Autodesk Inventor part; units mm, degrees
ref_plane "YZ Plane" through (0, 0, 0) normal (1, 0, 0) x (0, 1, 0)
ref_plane "XZ Plane" through (0, 0, 0) normal (0, 1, 0) x (-1, 0, 0)
ref_plane "XY Plane" through (0, 0, 0) normal (0, 0, 1) x (1, 0, 0)
sketch "Эскиз1" plane through (0, 0, 0) normal (0, 0, 1) x (1, 0, 0)
  circle A0 centre (0, 0) radius 11
  circle A1 centre (0, 0) radius 7.5
  circle A2 centre (-7.5, 0) radius 1.5
  circle A3 centre (0, -7.5) radius 1.5
  circle A4 centre (7.5, 0) radius 1.5
  circle A5 centre (0, 7.5) radius 1.5
  circle A6 centre (0, 0) radius 3
  dimension "d1" = 15
  dimension "d0" = 22
  dimension "d2" = 3
  dimension "d5" = 360
  dimension "d7" = 6
extrude "Выдавливание1" add sketch "Эскиз1" along normal blind 3 contours A0 | A4 A1 A3 A2 A5
sketch "Эскиз2" plane through (0, 0, 3) normal (0, 0, 1) x (1, 0, 0)
  circle A0 centre (0, 0) radius 4.5
  circle A1 centre (0, 0) radius 11
  circle A2 centre (0, 7.5) radius 1.5
  circle A3 centre (-7.5, 0) radius 1.5
  circle A4 centre (0, -7.5) radius 1.5
  circle A5 centre (0, 0) radius 3
  circle A6 centre (7.5, 0) radius 1.5
  dimension "d10" = 9
extrude "Выдавливание2" add sketch "Эскиз2" along normal blind 9 contours A0
fillet "Сопряжение1" radius 0.5 2 edges at (-11, 0, 3) (-4.5, 0, 3)
chamfer "Фаска1" distance 0.5 angle 45 2 edges at (-4.5, 0, 12) (-3, 0, 12)
properties part number "МУФТА НА ВАЛ"
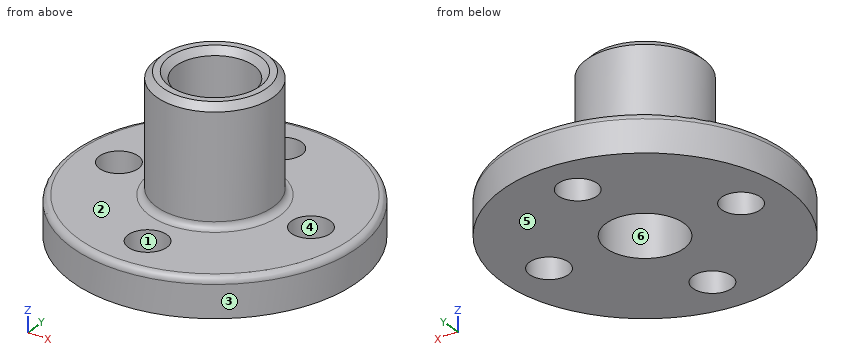
Check sheet for the modelled part. Datum: model origin and axes. Units: mm. Face numbers are marked on the shaded views. A direction names the side the tool comes from. Round coordinates to 2 decimals unless told otherwise and drop trailing zeros. Order: outer loops, then holes, each group sorted by start corner. A loop starts at its lowest first (then second) coordinate and runs counter-clockwise, first axis right, second up. Notation, with made-up numbers: (4.5, 43.25) -> (58.5, 43.25) arc R30 cw to (58.5, 69.25) -> close; hole circle Ø10 at (62.5, 43). An arc over 180 degrees is marked (long way). Use CSV: the item, a comma, the result in double quotes.
(1) Cross-section at A-A (x = 0). Record the boundary of the cut face in (y, z), and give its area (3 significant figures).
Worked out:
outline,"(-11, 0) -> (-9, 0) -> (-9, 3) -> (-10.5, 3) arc R0.5 ccw to (-11, 2.5) -> close; (-6, 0) -> (-3, 0) -> (-3, 11.5) -> (-3.5, 12) -> (-4, 12) -> (-4.5, 11.5) -> (-4.5, 3.5) arc R0.5 cw to (-5, 3) -> (-6, 3) -> close; (3, 0) -> (6, 0) -> (6, 3) -> (5, 3) arc R0.5 cw to (4.5, 3.5) -> (4.5, 11.5) -> (4, 12) -> (3.5, 12) -> (3, 11.5) -> close; (9, 0) -> (11, 0) -> (11, 2.5) arc R0.5 ccw to (10.5, 3) -> (9, 3) -> close"
area,"56.5 mm²"
(2) Draft check along Y on the marked faces 3, 4, 5 and 6. Enter one of: pulls with the +Y half, pulls with the -Y half, needs draft (parallel to the pull), parting line crosses it, or undercut.
Worked out:
face 3,"parting line crosses it"
face 4,"undercut"
face 5,"needs draft"
face 6,"undercut"
(3) Tool access check on the marked faces 1 and 2. Record the directions out of +Z, -Z, +X, -X, +Y, -Y that give a thin tool (end or side, any length) a straight path to the whole face; none if there is none.
Worked out:
face 1,"+Z, -Z"
face 2,"+Z"
(4) Material ranges on line 1 along Y through (x, z) = (0, 2.05); line 2 along Y through (x, z) = (0, 8.5); line 3 along Z through (x, y) = (-8.5, 4.75), recorded low to high. Write a range as from..to.
Worked out:
line 1,"-11..-9, -6..-3, 3..6, 9..11"
line 2,"-4.5..-3, 3..4.5"
line 3,"0..3"
(5) Depth check by flat-ended pin: pin 1 (4 mm diameter, centred on x = 0, y = 7.5, fed in from +Z); pin 2 (2 mm diameter, centred on x = 1, z = 7.5, fed in from +Y); pin 3 (2 mm diameter, centred on y = 3, z = 7.5, fed in from -X). Enter the tip coordinate at first touch or a pass-through.
Worked out:
pin 1,"z = 3"
pin 2,"y = 4.5"
pin 3,"x = -4.03"
(6) Cross-section at B-B (z = 1.5). Record the boundary of the cut face in (x, y).
Worked out:
outline,"circle Ø22 at (0, 0); hole circle Ø3 at (-7.5, 0); hole circle Ø6 at (0, 0); hole circle Ø3 at (0, -7.5); hole circle Ø3 at (0, 7.5); hole circle Ø3 at (7.5, 0)"
(7) Cross-section at C-C (z = 9.75). Record the boundary of the cut face in (x, y), and give its area (3 significant figures).
Worked out:
outline,"circle Ø9 at (0, 0); hole circle Ø6 at (0, 0)"
area,"35.3 mm²"
